Drawing for the job (mm, zero at the part's lowest x, y, z). A direction names the side the tool comes from. Coordinates: 2 decimals unless noted, no trailing zeros. Order: outer loops, then holes, each group sorted by start corner. A loop starts at its lowest first (then second) coordinate and runs counter-clockwise, first axis right, second up.
1) Cut at D-D (x = 5). List the corners of the cut face in (y, z), and give its area (3 significant figures).
2) Cut at A-A (x = 10). List the corners of the cut face in (y, z).
3) Cut at C-C (z = 8.5). List the corners of the cut face in (x, y), and give its area (3 significant figures).
4) Wall check: L1, parallel to Y at x = 12, z = 4; L2, parallel to Z at x = 19.25, y = 25.5; L3, parallel to Y at x = 10, z = 3.5. Give the ranges that are in metal, low to high.
5) Cut at B-B (y = 10). List the corners of the cut face in (x, z).
6) Pin check, flat tips, straight feed: pin 1 Ø1 at (y, z) = (26.5, 7.5) entering from -X; pin 2 Ø5 at (x, z) = (13, 7.5) entering from +Y; pin 3 Ø6 at (x, y) = (5, 23) entering from +Z. Stop position of each tip, or through.
7) Mould opens along Y. For the marked faces 1, 2, 3 and 4 say: +Y half, -Y half, draft (parallel to the pull), parting line (faces both ways), or undercut.
8) Tool access for the marked faces 5 and 6: list every direction of +Z, -Z, +X, -X, +Y, -Y with a clear straight run to the whole face (end or side of a thin tool).
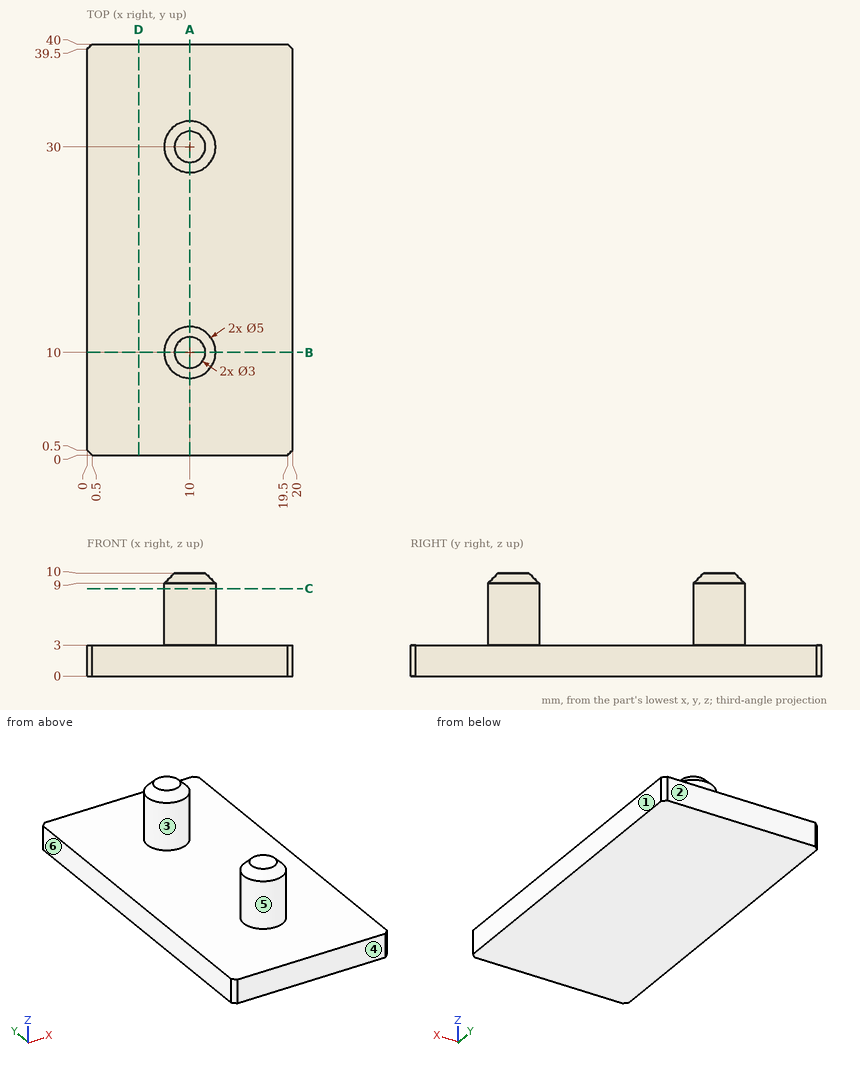
Geometry check:
1. outline: (0, 0) - (40, 0) - (40, 3) - (0, 3) - close
1. area: 120 mm2
2. outline: (0, 0) - (40, 0) - (40, 3) - (32.5, 3) - (32.5, 9) - (31.5, 10) - (28.5, 10) - (27.5, 9) - (27.5, 3) - (12.5, 3) - (12.5, 9) - (11.5, 10) - (8.5, 10) - (7.5, 9) - (7.5, 3) - (0, 3) - close
3. outline: circle Ø5 at (10, 10); circle Ø5 at (10, 30)
3. area: 39.3 mm2
4. L1: y = 8.5 to 11.5, 28.5 to 31.5
4. L2: z = 0 to 3
4. L3: y = 7.5 to 12.5, 27.5 to 32.5
5. outline: (0, 0) - (20, 0) - (20, 3) - (12.5, 3) - (12.5, 9) - (11.5, 10) - (8.5, 10) - (7.5, 9) - (7.5, 3) - (0, 3) - close
6. pin 1: passes through
6. pin 2: stops at y = 32.45
6. pin 3: stops at z = 3
7. face 1: draft
7. face 2: +Y half
7. face 3: undercut
7. face 4: -Y half
8. face 5: +Z
8. face 6: +Z, -Z, -X, +Y, -Y
